```python
from build123d import *

# Parameters (mm, degrees)
SKETCH2_W           = 150
SKETCH2_H           = 150
BOSS_EXTRUDE1_DEPTH = 5
SKETCH3_R           = 5
BOSS_EXTRUDE2_DEPTH = 20
SKETCH4_R           = 10
CUT_EXTRUDE1_DEPTH  = 108.935165725
SKETCH5_R           = 5.5
CUT_EXTRUDE2_DEPTH  = 20
FILLET1_R           = 10
SKETCH6_R           = 5
BOSS_EXTRUDE3_DEPTH = 5
SKETCH8_R           = 10
SKETCH8_R_2         = 5.5
CUT_EXTRUDE3_DEPTH  = 5
SKETCH9_R           = 2
SKETCH9_R_2         = 5.5
CUT_EXTRUDE4_DEPTH  = 5
SKETCH10_W          = 20
SKETCH10_H          = 20
CUT_EXTRUDE5_DEPTH  = 10


with BuildPart() as part:
    # Sketch2 → Boss-Extrude1 (new body)
    with BuildSketch(Plane(origin=(0, 0, 0), x_dir=(1, 0, 0), z_dir=(0, 1, 0))):
        Rectangle(SKETCH2_W, SKETCH2_H)
    extrude(amount=BOSS_EXTRUDE1_DEPTH)

    # Sketch3 → Boss-Extrude2 (add)
    with BuildSketch(Plane(origin=(0, 5, 0), x_dir=(1, 0, 0), z_dir=(0, 1, 0))):
        with Locations(Location((50, 50, 0), (0, 0, 270))):
            Circle(SKETCH3_R)
        with Locations(Location((50, -50, 0), (0, 0, 270))):
            Circle(SKETCH3_R)
        with Locations(Location((-50, -50, 0), (0, 0, 270))):
            Circle(SKETCH3_R)
        with Locations(Location((-50, 50, 0), (0, 0, 270))):
            Circle(SKETCH3_R)
    extrude(amount=BOSS_EXTRUDE2_DEPTH)

    # Sketch4 → Cut-Extrude1 (cut, through all)
    with BuildSketch(Plane(origin=(0, 5, 0), x_dir=(1, 0, 0), z_dir=(0, 1, 0))):
        with Locations(Location((0, 0, 0), (0, 0, 270))):
            Circle(SKETCH4_R)
    extrude(amount=-CUT_EXTRUDE1_DEPTH, mode=Mode.SUBTRACT)

    # Sketch5 → Cut-Extrude2 (cut)
    with BuildSketch(Plane(origin=(0, 5, 0), x_dir=(1, 0, 0), z_dir=(0, 1, 0))):
        with Locations(Location((-60, 0, 0), (0, 0, 270))):
            Circle(SKETCH5_R)
    extrude(amount=-CUT_EXTRUDE2_DEPTH, mode=Mode.SUBTRACT)

    # Fillet1
    fillet1_edges = [part.edges().sort_by_distance(p)[0] for p in [
        (75, 2.5, 75),
        (-75, 2.5, 75),
        (-75, 2.5, -75),
        (75, 2.5, -75),
    ]]
    fillet(fillet1_edges, radius=FILLET1_R)

    # Sketch6 → Boss-Extrude3 (add)
    with BuildSketch(Plane(origin=(0, 25, 0), x_dir=(1, 0, 0), z_dir=(0, 1, 0))):
        with BuildLine():
            Line((65, 75), (-65, 75))
            ThreePointArc((-65, 75), (-72.071067812, 72.071067812), (-75, 65))
            Line((-75, 65), (-75, -65))
            ThreePointArc((-75, -65), (-72.071067812, -72.071067812), (-65, -75))
            Line((-65, -75), (65, -75))
            ThreePointArc((65, -75), (72.071067812, -72.071067812), (75, -65))
            Line((75, -65), (75, 65))
            ThreePointArc((75, 65), (72.071067812, 72.071067812), (65, 75))
        make_face()
        with Locations(Location((-50, 50, 0), (0, 0, 270))):
            Circle(SKETCH6_R, mode=Mode.SUBTRACT)
        with Locations(Location((-50, 50, 0), (0, 0, 270))):
            Circle(SKETCH6_R)
    extrude(amount=BOSS_EXTRUDE3_DEPTH)

    # Sketch8 → Cut-Extrude3 (cut)
    with BuildSketch(Plane.XZ.offset(-25)):
        with Locations(Location((0, 0, 0), (0, 0, 90))):
            Circle(SKETCH8_R)
        with Locations(Location((-60, 0, 0), (0, 0, 90))):
            Circle(SKETCH8_R_2)
    extrude(amount=-CUT_EXTRUDE3_DEPTH, mode=Mode.SUBTRACT)

    # Sketch9 → Cut-Extrude4 (cut)
    with BuildSketch(Plane(origin=(0, 30, 0), x_dir=(1, 0, 0), z_dir=(0, 1, 0))):
        with Locations(Location((-47.448854634, 12.551145366, 0), (0, 0, 270))):
            Circle(SKETCH9_R)
        with Locations(Location((-60, 0, 0), (0, 0, 270))):
            Circle(SKETCH9_R_2)
        with Locations(Location((-47.448854634, -12.551145366, 0), (0, 0, 270))):
            Circle(SKETCH9_R)
        with Locations(Location((-72.551145366, -12.551145366, 0), (0, 0, 270))):
            Circle(SKETCH9_R)
        with Locations(Location((-72.551145366, 12.551145366, 0), (0, 0, 270))):
            Circle(SKETCH9_R)
    extrude(amount=-CUT_EXTRUDE4_DEPTH, mode=Mode.SUBTRACT)

    # Sketch10 → Cut-Extrude5 (cut)
    with BuildSketch(Plane(origin=(0, 30, 0), x_dir=(1, 0, 0), z_dir=(0, 1, 0))):
        with Locations((-65, 65)):
            Rectangle(SKETCH10_W, SKETCH10_H)
        with Locations((65, 65)):
            Rectangle(SKETCH10_W, SKETCH10_H)
        with Locations((65, -65)):
            Rectangle(SKETCH10_W, SKETCH10_H)
        with Locations((-65, -65)):
            Rectangle(SKETCH10_W, SKETCH10_H)
    extrude(amount=-CUT_EXTRUDE5_DEPTH, mode=Mode.SUBTRACT)


solid = part.part
```
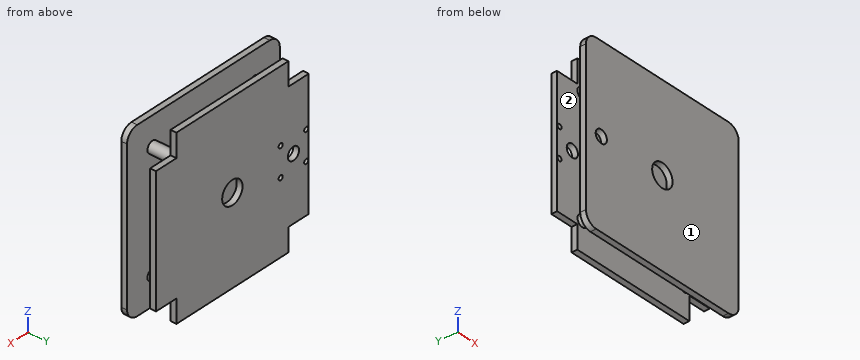
Model file for the job. Use its own axes, mm. Face numbers are marked on the shaded views. A direction names the side the tool comes from. Coordinates: 2 decimals unless noted, no trailing zeros. Loops run counter-clockwise (first coordinate to the right, second up) from the corner with the lowest first, then second, coordinate; pieces in that order, holes last. Notation, with made-up numbers: M 24,-4.5 L 56,-4.5 A16 cw 56,9.5 Z; hole C 37,79.5 d3. An arc over 180 degrees is marked long. Use CSV: the item, a comma, the result in double quotes. Start each with the question number.
1. Flat gauge pins, fed straight in: pin 1 (4 mm diameter, centred on x = -60, y = 27.5, fed in from -Z); pin 2 (1.5 mm diameter, centred on x = -62.5, y = 26.5, fed in from +Z); pin 3 (6 mm diameter, centred on y = 15, z = -47.5, fed in from +X). Where does each tip first touch, or does it go through?
2. Band-saw the part on A-A, the plane z = 21.5. List the corners of the cut face in (x, y).
3. Tool access for the marked faces 1 and 2: list every direction of +Z, -Z, +X, -X, +Y, -Y with a clear straight run to the whole face (end or side of a thin tool).
4. Band-saw the part on B-B, the plane x = 0. List the corners of the cut face in (y, z).
5. Probe probe 1 along X at (y, z) = (3.6, 0); probe 2 along Y at (x, z) = (-48, -37.5); probe 3 along Y at (x, z) = (-58.5, -65). List the from-to ranges inside material, lowest first. Write a range as [from, to].
6. Band-saw the part on C-C, the plane z = -50. List the corners of the cut face in (x, y), then the cut area to 3 significant figures.
7. Band-saw the part on D-D, the plane x = 50. List the corners of the cut face in (y, z), then the cut area to 3 significant figures.
Entries:
1,pin 1,"stops at z = -55"
1,pin 2,"stops at z = 55"
1,pin 3,"stops at x = 55"
2,outline,"M -75,0 L 75,0 L 75,5 L -75,5 Z; M -75,25 L 75,25 L 75,30 L -75,30 Z"
3,face 1,"+Z, -Z, +X, -X, -Y"
3,face 2,"none"
4,outline,"M 0,-75 L 5,-75 L 5,-10 L 0,-10 Z; M 0,10 L 5,10 L 5,75 L 0,75 Z; M 25,-75 L 30,-75 L 30,-10 L 25,-10 Z; M 25,10 L 30,10 L 30,75 L 25,75 Z"
5,probe 1,"x = [-75, -65.5], [-54.5, -10], [10, 75]"
5,probe 2,"y = [0, 5], [25, 30]"
5,probe 3,"y = [0, 5]"
6,outline,"M -75,0 L 75,0 L 75,5 L 55,5 L 55,25 L 75,25 L 75,30 L -75,30 L -75,25 L -55,25 L -55,5 L -75,5 Z; hole M -45,5 L 45,5 L 45,25 L -45,25 Z"
6,area,"1,900 mm2"
7,outline,"M 0,-75 L 5,-75 L 5,-55 L 25,-55 L 25,-75 L 30,-75 L 30,75 L 25,75 L 25,55 L 5,55 L 5,75 L 0,75 Z; hole M 5,-45 L 25,-45 L 25,45 L 5,45 Z"
7,area,"1,900 mm2"
